For this review, take the finished solid that the model builds, in its own axes (mm). Face numbers are marked on the shaded views. Coordinates: 2 decimals unless noted, no trailing zeros. Loops run counter-clockwise (first coordinate to the right, second up) from the corner with the lowest first, then second, coordinate; pieces in that order, holes last. Notation, with made-up numbers: (68, 21.5) - (123, 21.5) arc R19 cw to (123, 55.5) - close; hole circle Ø6 at (61.25, -11.5). An arc over 180 degrees is marked (long way). Use one line per item in the form item = value. Start each with the question number.
1. To check wall thickness, follow probe 1 along Y at (x, z) = (65.5, 47.2); probe 2 along Y at (x, z) = (210, 47.05); probe 3 along X at (y, z) = (-49, 40.75). State the ranges of each line that lie inside material, in increasing order.
2. For pin 1 Ø3 at (x, z) = (149, 45.5) entering from -Y; pin 2 Ø2.5 at (x, z) = (167, 41.5) entering from +Y; pin 3 Ø10 at (x, y) = (156.5, 37.5) entering from -Z, all flat-tipped, find the tip position at first contact; note any pin that passes through.
3. Add section A-A on x = 175.5. Give the boundary of the cut face in (y, z), and give its area (3 significant figures).
4. Add section C-C on x = 140. Give the boundary of the cut face in (y, z), and give its area (3 significant figures).
5. Draft analysis for pull direction Y (two halves, no side actions). For the marked faces 1 and 2, state which applies: +Y half, -Y half, draft (parallel to the pull), parting line (faces both ways), or undercut.
6. Add section D-D on y = 4. Give the boundary of the cut face in (x, z), and give its area (3 significant figures).
7. Add section B-B on z = 40.5. Give the boundary of the cut face in (x, y), and give its area (3 significant figures).
```python
from build123d import *
from build123d.topology import SkipClean

# Parameters (mm, degrees)
MAIN_PROFILE_SKETCH_R       = 3.4
MAIN_PROFILE_SKETCH_R_2     = 1.7
MAIN_EXTRUSION_DEPTH        = 3.5
DETAIL_PROFILE_2_SKETCH_R   = 5.3
DETAIL_PROFILE_2_SKETCH_R_2 = 1.7
DETAIL_EXTRUSION_2_DEPTH    = 0.5
DETAIL_PROFILE_3_SKETCH_W   = 85.5
DETAIL_PROFILE_3_SKETCH_H   = 3
DETAIL_EXTRUSION_3_DEPTH    = 0.2
DETAIL_PROFILE_4_SKETCH_W   = 85.5
DETAIL_PROFILE_4_SKETCH_H   = 3
DETAIL_EXTRUSION_4_DEPTH    = 7.8


with BuildPart() as part:
    # Main Profile Sketch → Main Extrusion (new body)
    with BuildSketch(Plane.XY.offset(48.5)):
        with BuildLine():
            Line((55, -55), (70.126602828, -55))
            ThreePointArc((70.126602828, -55), (75, -57.5), (79.873397172, -55))
            Line((79.873397172, -55), (204, -55))
            ThreePointArc((204, -55), (210, -58), (216, -55))
            Line((216, -55), (220, -55))
            Line((220, -55), (220, 55))
            Line((220, 55), (216, 55))
            ThreePointArc((216, 55), (210, 58), (204, 55))
            Line((204, 55), (79.873397172, 55))
            ThreePointArc((79.873397172, 55), (75, 57.5), (70.126602828, 55))
            Line((70.126602828, 55), (55, 55))
            Line((55, 55), (55, -55))
        make_face()
        with Locations((75, -51.5)):
            Circle(MAIN_PROFILE_SKETCH_R, mode=Mode.SUBTRACT)
        with Locations((65.5, -43.5)):
            Circle(MAIN_PROFILE_SKETCH_R_2, mode=Mode.SUBTRACT)
        with Locations((70, -36.5)):
            Circle(MAIN_PROFILE_SKETCH_R_2, mode=Mode.SUBTRACT)
        with Locations((79.5, -43.5)):
            Circle(MAIN_PROFILE_SKETCH_R_2, mode=Mode.SUBTRACT)
        with Locations((120.5, -43.5)):
            Circle(MAIN_PROFILE_SKETCH_R_2, mode=Mode.SUBTRACT)
        with Locations((134.5, -43.5)):
            Circle(MAIN_PROFILE_SKETCH_R_2, mode=Mode.SUBTRACT)
        with Locations((65.5, -10.5)):
            Circle(MAIN_PROFILE_SKETCH_R_2, mode=Mode.SUBTRACT)
        with Locations((79.5, -10.5)):
            Circle(MAIN_PROFILE_SKETCH_R_2, mode=Mode.SUBTRACT)
        with Locations((120.5, -10.5)):
            Circle(MAIN_PROFILE_SKETCH_R_2, mode=Mode.SUBTRACT)
        with Locations((134.5, -10.5)):
            Circle(MAIN_PROFILE_SKETCH_R_2, mode=Mode.SUBTRACT)
        with Locations((175.5, -43.5)):
            Circle(MAIN_PROFILE_SKETCH_R_2, mode=Mode.SUBTRACT)
        with Locations((210, -50.5)):
            Circle(MAIN_PROFILE_SKETCH_R_2, mode=Mode.SUBTRACT)
        with Locations((184, -34)):
            Circle(MAIN_PROFILE_SKETCH_R_2, mode=Mode.SUBTRACT)
        with Locations((216, -34)):
            Circle(MAIN_PROFILE_SKETCH_R_2, mode=Mode.SUBTRACT)
        with Locations((175.5, -10.5)):
            Circle(MAIN_PROFILE_SKETCH_R_2, mode=Mode.SUBTRACT)
        with Locations((65.5, 10.5)):
            Circle(MAIN_PROFILE_SKETCH_R_2, mode=Mode.SUBTRACT)
        with Locations((79.5, 10.5)):
            Circle(MAIN_PROFILE_SKETCH_R_2, mode=Mode.SUBTRACT)
        with Locations((120.5, 10.5)):
            Circle(MAIN_PROFILE_SKETCH_R_2, mode=Mode.SUBTRACT)
        with Locations((134.5, 10.5)):
            Circle(MAIN_PROFILE_SKETCH_R_2, mode=Mode.SUBTRACT)
        with Locations((70, 36.5)):
            Circle(MAIN_PROFILE_SKETCH_R_2, mode=Mode.SUBTRACT)
        with Locations((65.5, 43.5)):
            Circle(MAIN_PROFILE_SKETCH_R_2, mode=Mode.SUBTRACT)
        with Locations((75, 51.5)):
            Circle(MAIN_PROFILE_SKETCH_R, mode=Mode.SUBTRACT)
        with Locations((79.5, 43.5)):
            Circle(MAIN_PROFILE_SKETCH_R_2, mode=Mode.SUBTRACT)
        with Locations((120.5, 43.5)):
            Circle(MAIN_PROFILE_SKETCH_R_2, mode=Mode.SUBTRACT)
        with Locations((134.5, 43.5)):
            Circle(MAIN_PROFILE_SKETCH_R_2, mode=Mode.SUBTRACT)
        with Locations((175.5, 10.5)):
            Circle(MAIN_PROFILE_SKETCH_R_2, mode=Mode.SUBTRACT)
        with Locations((182, 0)):
            Circle(MAIN_PROFILE_SKETCH_R_2, mode=Mode.SUBTRACT)
        with Locations((218, 0)):
            Circle(MAIN_PROFILE_SKETCH_R_2, mode=Mode.SUBTRACT)
        with Locations((175.5, 43.5)):
            Circle(MAIN_PROFILE_SKETCH_R_2, mode=Mode.SUBTRACT)
        with Locations((184, 34)):
            Circle(MAIN_PROFILE_SKETCH_R_2, mode=Mode.SUBTRACT)
        with Locations((216, 34)):
            Circle(MAIN_PROFILE_SKETCH_R_2, mode=Mode.SUBTRACT)
        with Locations((210, 50.5)):
            Circle(MAIN_PROFILE_SKETCH_R_2, mode=Mode.SUBTRACT)
    extrude(amount=-MAIN_EXTRUSION_DEPTH)

    # Detail Profile 2 Sketch → Detail Extrusion 2 (add)
    with BuildSketch(Plane.XY.offset(45)):
        with BuildLine():
            Line((55, -55), (70.126602828, -55))
            ThreePointArc((70.126602828, -55), (75, -57.5), (79.873397172, -55))
            Line((79.873397172, -55), (204, -55))
            ThreePointArc((204, -55), (210, -58), (216, -55))
            Line((216, -55), (220, -55))
            Line((220, -55), (220, 55))
            Line((220, 55), (216, 55))
            ThreePointArc((216, 55), (210, 58), (204, 55))
            Line((204, 55), (79.873397172, 55))
            ThreePointArc((79.873397172, 55), (75, 57.5), (70.126602828, 55))
            Line((70.126602828, 55), (55, 55))
            Line((55, 55), (55, -55))
        make_face()
        with Locations((75, -51.5)):
            Circle(DETAIL_PROFILE_2_SKETCH_R, mode=Mode.SUBTRACT)
        with Locations((65.5, -43.5)):
            Circle(DETAIL_PROFILE_2_SKETCH_R_2, mode=Mode.SUBTRACT)
        with Locations((70, -36.5)):
            Circle(DETAIL_PROFILE_2_SKETCH_R_2, mode=Mode.SUBTRACT)
        with Locations((79.5, -43.5)):
            Circle(DETAIL_PROFILE_2_SKETCH_R_2, mode=Mode.SUBTRACT)
        with Locations((120.5, -43.5)):
            Circle(DETAIL_PROFILE_2_SKETCH_R_2, mode=Mode.SUBTRACT)
        with Locations((134.5, -43.5)):
            Circle(DETAIL_PROFILE_2_SKETCH_R_2, mode=Mode.SUBTRACT)
        with Locations((65.5, -10.5)):
            Circle(DETAIL_PROFILE_2_SKETCH_R_2, mode=Mode.SUBTRACT)
        with Locations((79.5, -10.5)):
            Circle(DETAIL_PROFILE_2_SKETCH_R_2, mode=Mode.SUBTRACT)
        with Locations((120.5, -10.5)):
            Circle(DETAIL_PROFILE_2_SKETCH_R_2, mode=Mode.SUBTRACT)
        with Locations((134.5, -10.5)):
            Circle(DETAIL_PROFILE_2_SKETCH_R_2, mode=Mode.SUBTRACT)
        with Locations((175.5, -43.5)):
            Circle(DETAIL_PROFILE_2_SKETCH_R_2, mode=Mode.SUBTRACT)
        with Locations((210, -50.5)):
            Circle(DETAIL_PROFILE_2_SKETCH_R_2, mode=Mode.SUBTRACT)
        with Locations((184, -34)):
            Circle(DETAIL_PROFILE_2_SKETCH_R_2, mode=Mode.SUBTRACT)
        with Locations((216, -34)):
            Circle(DETAIL_PROFILE_2_SKETCH_R_2, mode=Mode.SUBTRACT)
        with Locations((175.5, -10.5)):
            Circle(DETAIL_PROFILE_2_SKETCH_R_2, mode=Mode.SUBTRACT)
        with Locations((65.5, 10.5)):
            Circle(DETAIL_PROFILE_2_SKETCH_R_2, mode=Mode.SUBTRACT)
        with Locations((79.5, 10.5)):
            Circle(DETAIL_PROFILE_2_SKETCH_R_2, mode=Mode.SUBTRACT)
        with Locations((120.5, 10.5)):
            Circle(DETAIL_PROFILE_2_SKETCH_R_2, mode=Mode.SUBTRACT)
        with Locations((134.5, 10.5)):
            Circle(DETAIL_PROFILE_2_SKETCH_R_2, mode=Mode.SUBTRACT)
        with Locations((70, 36.5)):
            Circle(DETAIL_PROFILE_2_SKETCH_R_2, mode=Mode.SUBTRACT)
        with Locations((65.5, 43.5)):
            Circle(DETAIL_PROFILE_2_SKETCH_R_2, mode=Mode.SUBTRACT)
        with Locations((75, 51.5)):
            Circle(DETAIL_PROFILE_2_SKETCH_R, mode=Mode.SUBTRACT)
        with Locations((79.5, 43.5)):
            Circle(DETAIL_PROFILE_2_SKETCH_R_2, mode=Mode.SUBTRACT)
        with Locations((120.5, 43.5)):
            Circle(DETAIL_PROFILE_2_SKETCH_R_2, mode=Mode.SUBTRACT)
        with Locations((134.5, 43.5)):
            Circle(DETAIL_PROFILE_2_SKETCH_R_2, mode=Mode.SUBTRACT)
        with Locations((175.5, 10.5)):
            Circle(DETAIL_PROFILE_2_SKETCH_R_2, mode=Mode.SUBTRACT)
        with Locations((182, 0)):
            Circle(DETAIL_PROFILE_2_SKETCH_R_2, mode=Mode.SUBTRACT)
        with Locations((218, 0)):
            Circle(DETAIL_PROFILE_2_SKETCH_R_2, mode=Mode.SUBTRACT)
        with Locations((175.5, 43.5)):
            Circle(DETAIL_PROFILE_2_SKETCH_R_2, mode=Mode.SUBTRACT)
        with Locations((184, 34)):
            Circle(DETAIL_PROFILE_2_SKETCH_R_2, mode=Mode.SUBTRACT)
        with Locations((216, 34)):
            Circle(DETAIL_PROFILE_2_SKETCH_R_2, mode=Mode.SUBTRACT)
        with Locations((210, 50.5)):
            Circle(DETAIL_PROFILE_2_SKETCH_R_2, mode=Mode.SUBTRACT)
    extrude(amount=-DETAIL_EXTRUSION_2_DEPTH)

    # Detail Profile 3 Sketch → Detail Extrusion 3 (add)
    with SkipClean():  # the faces are left unmerged after this step: merging them gives an invalid solid
        with BuildSketch(Plane.XY.offset(44.5)):
            with BuildLine():
                Line((58, -48.5), (70.630789545, -48.5))
                ThreePointArc((70.630789545, -48.5), (69.938043095, -49.929461145), (69.7, -51.5))
                Line((69.7, -51.5), (58, -51.5))
                Line((58, -51.5), (58, -48.5))
            make_face()
            with BuildLine():
                Line((79.369210455, -48.5), (80, -48.5))
                Line((80, -48.5), (80, -49.742160417))
                ThreePointArc((80, -49.742160417), (79.725596974, -49.100263923), (79.369210455, -48.5))
            make_face()
            with Locations((145.75, -50)):
                Rectangle(DETAIL_PROFILE_3_SKETCH_W, DETAIL_PROFILE_3_SKETCH_H)
            with BuildLine():
                Line((58, 51.5), (58, 48.5))
                Line((58, 48.5), (70.630789545, 48.5))
                ThreePointArc((70.630789545, 48.5), (69.938043095, 49.929461145), (69.7, 51.5))
                Line((69.7, 51.5), (58, 51.5))
            make_face()
            with BuildLine():
                Line((80, 49.742160417), (80, 48.5))
                Line((80, 48.5), (79.369210455, 48.5))
                ThreePointArc((79.369210455, 48.5), (79.725596974, 49.100263923), (80, 49.742160417))
            make_face()
            with Locations((145.75, 50)):
                Rectangle(DETAIL_PROFILE_3_SKETCH_W, DETAIL_PROFILE_3_SKETCH_H)
        extrude(amount=-DETAIL_EXTRUSION_3_DEPTH)

    # Detail Profile 4 Sketch → Detail Extrusion 4 (add)
    with SkipClean():  # the faces are left unmerged after this step: merging them gives an invalid solid
        with BuildSketch(Plane.XY.offset(44.3)):
            with BuildLine():
                Line((58, -48.5), (73.625227292, -48.5))
                ThreePointArc((73.625227292, -48.5), (72.222703658, -49.717691096), (71.7, -51.5))
                Line((71.7, -51.5), (58, -51.5))
                Line((58, -51.5), (58, -48.5))
            make_face()
            with BuildLine():
                Line((80, -48.5), (80, -51.5))
                Line((80, -51.5), (78.3, -51.5))
                ThreePointArc((78.3, -51.5), (77.777296342, -49.717691096), (76.374772708, -48.5))
                Line((76.374772708, -48.5), (80, -48.5))
            make_face()
            with Locations((145.75, -50)):
                Rectangle(DETAIL_PROFILE_4_SKETCH_W, DETAIL_PROFILE_4_SKETCH_H)
            with BuildLine():
                Line((58, 51.5), (58, 48.5))
                Line((58, 48.5), (73.625227292, 48.5))
                ThreePointArc((73.625227292, 48.5), (72.222703658, 49.717691096), (71.7, 51.5))
                Line((71.7, 51.5), (58, 51.5))
            make_face()
            with BuildLine():
                Line((78.3, 51.5), (80, 51.5))
                Line((80, 51.5), (80, 48.5))
                Line((80, 48.5), (76.374772708, 48.5))
                ThreePointArc((76.374772708, 48.5), (77.777296342, 49.717691096), (78.3, 51.5))
            make_face()
            with Locations((145.75, 50)):
                Rectangle(DETAIL_PROFILE_4_SKETCH_W, DETAIL_PROFILE_4_SKETCH_H)
        extrude(amount=-DETAIL_EXTRUSION_4_DEPTH)


solid = part.part
```
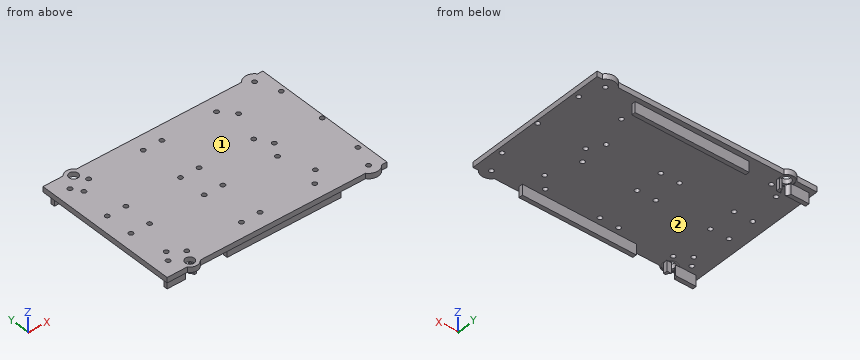
Conclusion:
q1.probe_1 = -55 to -45.2, -41.8 to -12.2, -8.8 to 8.8, 12.2 to 41.8, 45.2 to 55
q1.probe_2 = -58 to -52.2, -48.8 to 48.8, 52.2 to 58
q1.probe_3 = 58 to 72.85, 77.15 to 80, 103 to 188.5
q2.pin_1 = -55
q2.pin_2 = 51.5
q2.pin_3 = 44.5
q3.outline = (-55, 44.5) - (-51.5, 44.5) - (-51.5, 36.5) - (-48.5, 36.5) - (-48.5, 44.5) - (-45.2, 44.5) - (-45.2, 48.5) - (-55, 48.5) - close; (-41.8, 44.5) - (-12.2, 44.5) - (-12.2, 48.5) - (-41.8, 48.5) - close; (-8.8, 44.5) - (8.8, 44.5) - (8.8, 48.5) - (-8.8, 48.5) - close; (12.2, 44.5) - (41.8, 44.5) - (41.8, 48.5) - (12.2, 48.5) - close; (45.2, 44.5) - (48.5, 44.5) - (48.5, 36.5) - (51.5, 36.5) - (51.5, 44.5) - (55, 44.5) - (55, 48.5) - (45.2, 48.5) - close
q3.area = 434 mm^2
q4.outline = (-55, 44.5) - (-51.5, 44.5) - (-51.5, 36.5) - (-48.5, 36.5) - (-48.5, 44.5) - (48.5, 44.5) - (48.5, 36.5) - (51.5, 36.5) - (51.5, 44.5) - (55, 44.5) - (55, 48.5) - (-55, 48.5) - close
q4.area = 488 mm^2
q5.face_1 = draft
q5.face_2 = undercut
q6.outline = (55, 44.5) - (220, 44.5) - (220, 48.5) - (55, 48.5) - close
q6.area = 660 mm^2
q7.outline = (58, -51.5) - (71.7, -51.5) arc R3.3 cw to (73.63, -48.5) - (58, -48.5) - close; (58, 48.5) - (73.63, 48.5) arc R3.3 cw to (71.7, 51.5) - (58, 51.5) - close; (76.37, -48.5) arc R3.3 cw to (78.3, -51.5) - (80, -51.5) - (80, -48.5) - close; (76.37, 48.5) - (80, 48.5) - (80, 51.5) - (78.3, 51.5) arc R3.3 cw to start; (103, -51.5) - (188.5, -51.5) - (188.5, -48.5) - (103, -48.5) - close; (103, 48.5) - (188.5, 48.5) - (188.5, 51.5) - (103, 51.5) - close
q7.area = 612 mm^2
